from build123d import *

# Parameters (mm, degrees)
F2_R      = 102
F3_DEPTH  = 5
F4_R      = 1
F5_W      = 9
F5_H      = 18
F5_R      = 2.5
F7_DEPTH  = 12.5
F6_W      = 9
F6_H      = 18
F6_R      = 1.75
F8_DEPTH  = 12.5
F9_W      = 250
F9_H      = 100
F10_DEPTH = 150
F11_R     = 2
F12_R     = 2


with BuildPart() as f1:
    # F0 (on Front) → F1 (revolve)
    with BuildSketch(Plane.XZ):
        with BuildLine():
            Line((-107.5, -3), (-96.5, -3))
            Line((-96.5, -3), (-96.5000625723, 0))
            Line((-96.5000625723, 0), (-96.5002087619, 7.009))
            Line((-96.5002087619, 7.009), (-112.6502087619, 7.009))
            Line((-112.6502087619, 7.009), (-112.6502087619, 5.009))
            ThreePointArc((-112.6502087619, 5.009), (-110.3061458059, 0.2465201859), (-109.5, -5))
            Line((-109.5, -5), (-109.5, -11))
            Line((-109.5, -11), (-107.5, -11))
            Line((-107.5, -11), (-107.5, -3))
        make_face()
    revolve(axis=Axis((0, 0, -0.2650997043), (0, 0, 1)))

    # F2 (on Top) → F3 (cut)
    with BuildSketch(Plane.XY):
        Circle(F2_R)
    extrude(amount=F3_DEPTH, mode=Mode.SUBTRACT)

    # F4
    f4_edges = [f1.edges().sort_by_distance(p)[0] for p in [
        (109.5, 0, -11),
    ]]
    fillet(f4_edges, radius=F4_R)

    # F5 (on Front) → F7 (join, symmetric)
    with BuildSketch(Plane.XZ):
        with Locations((-112.2, -2)):
            Rectangle(F5_W, F5_H)
        with Locations((-112.2, -2)):
            Circle(F5_R, mode=Mode.SUBTRACT)
    extrude(amount=F7_DEPTH, both=True)

    # F6 (on Front) → F8 (join, symmetric)
    with BuildSketch(Plane.XZ):
        with Locations((112.2, -2)):
            Rectangle(F6_W, F6_H)
        with Locations((112.2, -2)):
            Circle(F6_R, mode=Mode.SUBTRACT)
    extrude(amount=F8_DEPTH, both=True)

    # F9 (on Front) → F10 (cut)
    with BuildSketch(Plane.XZ):
        with Locations((0.1239156971, -32.2915658355)):
            Rectangle(F9_W, F9_H)
    extrude(amount=-F10_DEPTH, mode=Mode.SUBTRACT)

    # F11
    f11_edges = [f1.edges().sort_by_distance(p)[0] for p in [
        (0, -102, 0),
    ]]
    fillet(f11_edges, radius=F11_R)

    # F12
    f12_edges = [f1.edges().sort_by_distance(p)[0] for p in [
        (116.7, -6.25, -11),
        (-116.7, -6.25, -11),
    ]]
    fillet(f12_edges, radius=F12_R)


solid = f1.part
Here's how the part is built. I have some questions about the finished solid (model axes, mm). A direction names the side the tool comes from. Give positions to 0.01 mm unless a question says otherwise; leave off trailing zeros. Order: outer loops, then holes, each group sorted by start corner. A loop starts at its lowest first (then second) coordinate and runs counter-clockwise, first axis right, second up. Notation, with made-up numbers: M 42,37.5 L 58,37.5 A13 ccw 58,51.5 Z; hole C -16,12 d10. An arc over 180 degrees is marked long. Answer as a JSON object with one key per item and string values. Group by question number.
1) Please list where these lines run through material, in increasing order: L1, parallel to X at y = -3, z = -2; L2, parallel to X at y = -8.25, z = -2; L3, parallel to Z at x = 17.5, y = -95. Write a range as [from, to].
2) I'm going to push flat-ended pins straight in: pin 1 Ø8 at (y, z) = (-20.5, -5) entering from -X; pin 2 Ø2.5 at (x, y) = (-114.5, -6.5) entering from +Z; pin 3 Ø5 at (y, z) = (-58.5, -7.5) entering from -X. Where does each tip first touch, or does it pass through?
3) We'd pull the mould along X, two halves only. Please class faces 1 (the cylindrical face through (-2.232, -109.477, -7.535)), 2 (the flat face through (-114, -12.5, -4)), 3 (the cylindrical face through (-114.2, -6.2, -3.5)): pulls with the +X half, pulls with the -X half, needs draft (parallel to the pull), parting line crosses it, or undercut.
4) Suppose I cut it at A-A, the plane x = 0. Write out the boundary of the cut face in (y, z).
5) On a 3-axis mill with a long thin cutter (end or side, diameter ignored), from which of +Z, -Z, +X, -X, +Y, -Y can I reach the whole of each face in a straight line? I mean faces 4 (the cylindrical face through (-2.364, -107.474, -6.944)), 5 (the flat face through (15, -96, 5)), 6 (the flat face through (113, -12.5, -4)). Say none if no direction works.
Results found:
{
 "1": {"L1": "[-116.7, -114.7], [-109.72, -96.45], [96.45, 110.45], [113.95, 116.7]", "L2": "[-116.7, -114.7], [-109.7, -96.15], [96.15, 110.45], [113.95, 116.7]", "L3": "[-3, 0], [5, 7.01]"},
 "2": {"pin 1": "x = -108.3", "pin 2": "z = 7", "pin 3": "x = -94.1"},
 "3": {"face 1": "parting line crosses it", "face 2": "needs draft", "face 3": "undercut"},
 "4": {"outline": "M -112.65,5.01 A17.48 cw -109.5,-5 L -109.5,-10 A1 ccw -108.5,-11 L -107.5,-11 L -107.5,-3 L -96.5,-3 L -96.5,0 L -100,0 A2 cw -102,2 L -102,5 L -96.5,5 L -96.5,7.01 L -112.65,7.01 Z"},
 "5": {"face 4": "-Z, +Y", "face 5": "+Y", "face 6": "-Z, +X, -Y"}
}
